```python
from build123d import *

# Parameters (mm, degrees)
ESBO_O1_W                          = 15
ESBO_O1_H                          = 50
RESSALTO_EXTRUS_O1_DEPTH           = 5
RESSALTO_EXTRUS_O1_2_DEPTH         = 5
ESBO_O1_4_W                        = 60
ESBO_O1_4_H                        = 50
ESBO_O1_4_W_2                      = 56
ESBO_O1_4_H_2                      = 46
RESSALTO_EXTRUS_O2_DEPTH           = 50
ESBO_O3_W                          = 50
ESBO_O3_H                          = 60
RESSALTO_EXTRUS_O3_DEPTH           = 2
FURO_ROSCADO_DE_G1_164_D           = 6.6
FURO_ROSCADO_DE_G1_164_CSINK_D     = 7.773
FURO_ROSCADO_DE_G1_164_CSINK_ANGLE = 90


with BuildPart() as part:
    # Esbo_o1 → Ressalto-extrus_o1 (new body)
    with BuildSketch(Plane(origin=(0, 0, 0), x_dir=(0, 1, 0), z_dir=(0, 0, 1))):
        with Locations((37.5, 0)):
            Rectangle(ESBO_O1_W, ESBO_O1_H)
    extrude(amount=RESSALTO_EXTRUS_O1_DEPTH)



with BuildPart() as body_2:
    # Esbo_o1 → Ressalto-extrus_o1 2 (new body)
    with BuildSketch(Plane(origin=(0, 0, 0), x_dir=(0, 1, 0), z_dir=(0, 0, 1))):
        with Locations((-37.5, 0)):
            Rectangle(ESBO_O1_W, ESBO_O1_H)
    extrude(amount=RESSALTO_EXTRUS_O1_2_DEPTH)


with BuildPart() as part_1:
    add(part.part)

    add(body_2.part)  # Ressalto-extrus_o2 merges body 2
    # Esbo_o1_4 → Ressalto-extrus_o2 (add)
    with BuildSketch(Plane(origin=(0, 0, 0), x_dir=(0, 1, 0), z_dir=(0, 0, 1))):
        Rectangle(ESBO_O1_4_W, ESBO_O1_4_H)
        Rectangle(ESBO_O1_4_W_2, ESBO_O1_4_H_2, mode=Mode.SUBTRACT)
    extrude(amount=RESSALTO_EXTRUS_O2_DEPTH)

    # Esbo_o3 → Ressalto-extrus_o3 (add)
    with BuildSketch(Plane.XY.offset(50)):
        Rectangle(ESBO_O3_W, ESBO_O3_H)
    extrude(amount=RESSALTO_EXTRUS_O3_DEPTH)

    # Furo roscado de G1_164 (through all)
    with Locations(Plane(origin=(0, 0, 5), x_dir=(0, -1, 0), z_dir=(0, 0, 1))):
        with Locations((37.5, 0), (-37.5, 0)):
            CounterSinkHole(FURO_ROSCADO_DE_G1_164_D / 2, FURO_ROSCADO_DE_G1_164_CSINK_D / 2, counter_sink_angle=FURO_ROSCADO_DE_G1_164_CSINK_ANGLE)


solid = part_1.part
```
Could you check a few things on this model? Use its own coordinates, in mm. A direction names the side the tool comes from. Coordinates: 2 decimals unless noted, no trailing zeros. Write each loop counter-clockwise with the first axis right and the second up, starting at its lowest first coordinate (ties: lowest second). Pieces come first, ordered by that corner, then holes. Notation, with made-up numbers: (30, 6.5) -> (78, 6.5) arc R37 cw to (78, 42.5) -> close; hole circle Ø11 at (-9.5, 43.5). An arc over 180 degrees is marked (long way). Return JSON: item names as keys, results as strings.
(1) Imagine slicing it at B-B, the plane x = 0. Please give me the cut outline in (y, z), then the cut area to 3 significant figures.
Numbers:
{"outline": "(-45, 0) -> (-40.8, 0) -> (-40.8, 4.41) -> (-41.39, 5) -> (-45, 5) -> close; (-34.2, 0) -> (-28, 0) -> (-28, 50) -> (28, 50) -> (28, 0) -> (34.2, 0) -> (34.2, 4.41) -> (33.61, 5) -> (30, 5) -> (30, 52) -> (-30, 52) -> (-30, 5) -> (-33.61, 5) -> (-34.2, 4.41) -> close; (40.8, 0) -> (45, 0) -> (45, 5) -> (41.39, 5) -> (40.8, 4.41) -> close", "area": "403 mm2"}
(2) Imagine slicing it at C-C, the plane z = 32. Please give me the cut outline in (x, y), then the cut area to 3 significant figures.
Numbers:
{"outline": "(-25, -30) -> (25, -30) -> (25, 30) -> (-25, 30) -> close; hole (-23, -28) -> (23, -28) -> (23, 28) -> (-23, 28) -> close", "area": "424 mm2"}
(3) I'm going to push flat-ended pins straight in: pin 1 (6 mm diameter, centred on x = -5.5, y = -19, fed in from -Z); pin 2 (8.5 mm diameter, centred on x = 0, y = -37.5, fed in from +Z); pin 3 (23 mm diameter, centred on x = 4, z = 20.5, fed in from +Y). Where does each tip first touch, or does it pass through?
Numbers:
{"pin 1": "stops at z = 50", "pin 2": "stops at z = 5", "pin 3": "stops at y = 30"}
(4) I need wall thicknesses on L1, parallel to Y at x = 0, z = 1.95; L2, parallel to X at y = -11, z = 17; L3, parallel to X at y = -37.5, z = 2.55. Which ranges of each line are inside material? Lowest first, please.
Numbers:
{"L1": "y = -45 to -40.8, -34.2 to -28, 28 to 34.2, 40.8 to 45", "L2": "x = -25 to -23, 23 to 25", "L3": "x = -25 to -3.3, 3.3 to 25"}
(5) Which directions (+Z, -Z, +X, -X, +Y, -Y) give clear straight access to the entire face, cutting with the end or side of a thin tool? Please do faces 1 (the flat face through (0, 30, 28)), 2 (the flat face through (23, 0, 25)), 3 (the flat face through (0, -43, 5)).
Numbers:
{"face 1": "+Z, +X, -X, +Y", "face 2": "-Z", "face 3": "+Z, +X, -X, -Y"}
(6) Imagine slicing it at D-D, the plane y = 27. Please give me the cut outline in (x, z).
Numbers:
{"outline": "(-25, 0) -> (-23, 0) -> (-23, 50) -> (23, 50) -> (23, 0) -> (25, 0) -> (25, 52) -> (-25, 52) -> close"}
(7) Imagine slicing it at A-A, the plane y = -37.5. Please give me the cut outline in (x, z), then the cut area to 3 significant figures.
Numbers:
{"outline": "(-25, 0) -> (-3.3, 0) -> (-3.3, 4.41) -> (-3.89, 5) -> (-25, 5) -> close; (3.3, 0) -> (25, 0) -> (25, 5) -> (3.89, 5) -> (3.3, 4.41) -> close", "area": "217 mm2"}
